Read the model definition and answer for the solid it produces. Units are mm, in the model's axes. Face numbers are marked on the shaded views. A direction names the side the tool comes from. Coordinates: 2 decimals unless noted, no trailing zeros. Loops run counter-clockwise (first coordinate to the right, second up) from the corner with the lowest first, then second, coordinate; pieces in that order, holes last. Notation, with made-up numbers: M -38,-38.5 L 1,-38.5 A33 cw 1,-9.5 Z; hole C 77.25,87.25 d8. An arc over 180 degrees is marked long. Put each result on its own line as item: value.
from build123d import *

# Parameters (mm, degrees)
BOSS_EXTRUDE1_DEPTH = 18.3896
FILLET1_R           = 1.1938
CHAMFER1_SIZE       = 0.254
CHAMFER2_SIZE       = 0.254


with BuildPart() as part:
    # Sketch1 → Boss-Extrude1 (new body)
    with BuildSketch(Plane.XY):
        Polygon((0, 10.089311424), (-8.7376, 5.044655712), (-8.7376, -5.044655712), (0, -10.089311424), (8.7376, -5.044655712), (8.7376, 5.044655712), align=None)
    extrude(amount=BOSS_EXTRUDE1_DEPTH)

    # Sketch2 → Cut-Revolve1 (revolve, cut)
    with BuildSketch(Plane(origin=(0, 0, 0), x_dir=(0, 0, -1), z_dir=(1, 0, 0))):
        Polygon((-18.3896, 11.453722848), (-18.3896, 8.7249), (-16.6624, 8.7249), (-16.296807061, 10.089311424), (-4.327992939, 10.089311424), (-3.9624, 8.7249), (0, 8.7249), (0, 11.453722848), align=None)
        with BuildLine():
            Line((-18.3896, 5.588), (-18.3896, 0))
            Line((-18.3896, 0), (0, 0))
            Line((0, 0), (0, 6.370416378))
            Line((0, 6.370416378), (-15.0622, 6.370416378))
            ThreePointArc((-15.0622, 6.370416378), (-15.241805122, 6.2960215), (-15.3162, 6.116416378))
            Line((-15.3162, 6.116416378), (-15.3162, 5.588))
            Line((-15.3162, 5.588), (-18.3896, 5.588))
        make_face()
    revolve(axis=Axis((0, 0, 0), (0, 0, 1)), mode=Mode.SUBTRACT)

    # Fillet1
    fillet1_edges = [part.edges().sort_by_distance(p)[0] for p in [
        (0, -8.7249, 18.3896),
    ]]
    fillet(fillet1_edges, radius=FILLET1_R)

    # Chamfer1
    chamfer1_edges = [part.edges().sort_by_distance(p)[0] for p in [
        (0, -8.7249, 0),
    ]]
    chamfer(chamfer1_edges, length=CHAMFER1_SIZE)

    # Chamfer2
    chamfer2_edges = [part.edges().sort_by_distance(p)[0] for p in [
        (0, -5.588, 18.3896),
        (0, -5.588, 15.3162),
    ]]
    chamfer(chamfer2_edges, length=CHAMFER2_SIZE)


solid = part.part
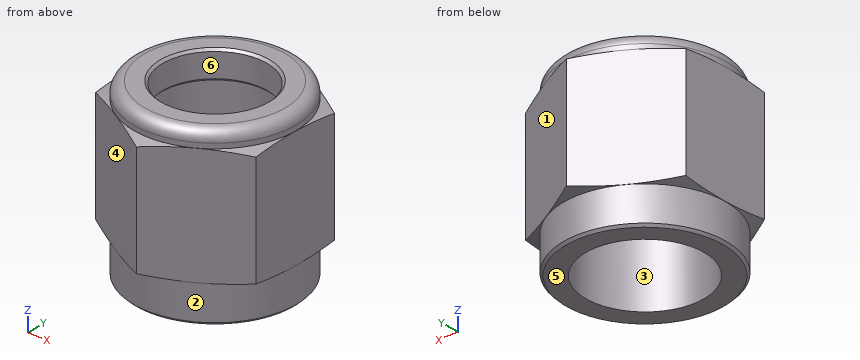
1) Find section B-B, the plane z = 5.25. Write down the section's boundary in (x, y), plus the area to 3 significant figures.
Answer list:
outline: M -8.74,-5.04 L 0,-10.09 L 8.74,-5.04 L 8.74,5.04 L 0,10.09 L -8.74,5.04 Z; hole C 0,0 d12.74
area: 137 mm^2
2) Determine the mould class of the marked faces 3, 4, 5 and 6 for opening direction Y: released by +Y, released by -Y, zero draft, split by the parting line, or undercut.
Answer list:
face 3: undercut
face 4: released by -Y
face 5: zero draft
face 6: undercut
3) Straight lines are drawn through the part: line 1 (X direction, y = 0, z = 16.8); line 2 (X direction, y = 0, z = 11.75). For each, find the intervals that lie inside material, in ascending order. Write a range as [from, to].
Answer list:
line 1: x = [-8.72, -5.59], [5.59, 8.72]
line 2: x = [-8.74, -6.37], [6.37, 8.74]
4) Find section C-C, the plane z = 2. Write down the section's boundary in (x, y), plus the area to 3 significant figures.
Answer list:
outline: C 0,0 d17.45; hole C 0,0 d12.74
area: 112 mm^2
5) Given pin 1 Ø3 at (x, z) = (-6.5, 6) entering from -Y, flat-ended and moving along its own axis, determine where the tip first touches the part or whether it passes through.
Answer list:
pin 1: stops at y = -7.2
6) Which of the six approach directions +Z, -Z, +X, -X, +Y, -Y give full straight-line access (tool end or side, diameter ignored) to the marked faces 1 and 2?
Answer list:
face 1: +Z, -Z, +X, +Y
face 2: -Z
